```python
from build123d import *

# Parameters (mm, degrees)
SKETCH3_W           = 8
SKETCH3_H           = 8
BOSS_EXTRUDE2_DEPTH = 15.2
SKETCH4_W           = 12
SKETCH4_H           = 12
BOSS_EXTRUDE3_DEPTH = 1


with BuildPart() as part:
    # Sketch1 → Revolve1 (revolve)
    with BuildSketch(Plane(origin=(0, 0, 0), x_dir=(0, 0, -1), z_dir=(1, 0, 0))):
        Polygon((-19.2, 0), (30.8, 0), (30.8, 5), (29.8, 5), (29.8, 4), (14.6, 4), (14.6, 3.5), (13.4, 3.5), (13.4, 4), (0, 4), (0, 2.5), (-15.4, 2.5), (-15.4, 2), (-16.2, 2), (-16.2, 2.5), (-19.2, 2.5), align=None)
    revolve(axis=Axis((0, 0, 19.2), (0, 0, -1)))

    # Sketch3 → Boss-Extrude2 (add)
    with BuildSketch(Plane.XY.offset(-29.8)):
        Rectangle(SKETCH3_W, SKETCH3_H)
    extrude(amount=BOSS_EXTRUDE2_DEPTH)

    # Sketch4 → Boss-Extrude3 (add)
    with BuildSketch(Plane(origin=(0, 0, -30.8), x_dir=(-1, 0, 0), z_dir=(0, 0, -1))):
        Rectangle(SKETCH4_W, SKETCH4_H)
    extrude(amount=-BOSS_EXTRUDE3_DEPTH)


solid = part.part
```
Here's how the part is built. I have some questions about the finished solid (model axes, mm). A direction names the side the tool comes from. Round coordinates to 2 decimals unless told otherwise and drop trailing zeros. Loops run counter-clockwise (first coordinate to the right, second up) from the corner with the lowest first, then second, coordinate; pieces in that order, holes last.
1. Suppose I cut it at A-A, the plane y = 0. Please give me the cut outline in (x, z), and give its area (3 significant figures).
Answers:
outline: (-6, -30.8) - (6, -30.8) - (6, -29.8) - (4, -29.8) - (4, -14.6) - (3.5, -14.6) - (3.5, -13.4) - (4, -13.4) - (4, 0) - (2.5, 0) - (2.5, 15.4) - (2, 15.4) - (2, 16.2) - (2.5, 16.2) - (2.5, 19.2) - (-2.5, 19.2) - (-2.5, 16.2) - (-2, 16.2) - (-2, 15.4) - (-2.5, 15.4) - (-2.5, 0) - (-4, 0) - (-4, -13.4) - (-3.5, -13.4) - (-3.5, -14.6) - (-4, -14.6) - (-4, -29.8) - (-6, -29.8) - close
area: 344 mm2
2. Will these pins go through, and if not, where does the flat tip stop? pin 1 (4 mm diameter, centred on x = 1.5, z = -22, fed in from -Y); pin 2 (1.5 mm diameter, centred on x = -4, z = 13, fed in from -Y); pin 3 (5 mm diameter, centred on y = 2, z = 5, fed in from -X); pin 4 (6 mm diameter, centred on x = 0.5, y = 2.5, fed in from +Z).
Answers:
pin 1: stops at y = -4
pin 2: passes through
pin 3: stops at x = -2.5
pin 4: stops at z = 19.2
3. If I drill on probe 1 along Z at (x, y) = (-1.25, 2); probe 2 along Y at (x, z) = (2.5, -27.5); probe 3 along Z at (x, y) = (5, 1.5), over which ranges is the centre line in solid material (lowest first)?
Answers:
probe 1: z = -30.8 to 15.4, 16.2 to 19.2
probe 2: y = -4 to 4
probe 3: z = -30.8 to -29.8
4. For faces 5 (the face through (4, 0, -22)), 6 (the face through (0, -4, -22)), 7 (the face through (2, -1, 15.4)), which set-ups out of +Z, -Z, +X, -X, +Y, -Y let a thin tool reach every point of the face, with its end or its side?
Answers:
face 5: +Z, +X, +Y, -Y
face 6: +Z, +X, -X, -Y
face 7: none
5. Suppose I cut it at C-C, the plane z = -5.5. Please give me the cut outline in (x, y), and give its area (3 significant figures).
Answers:
outline: circle Ø8 at (0, 0)
area: 50.3 mm2
6. Thinking about a two-plate mould opening in Z: for faces 1 (the face through (2, 1, 16.2)), 2 (the face through (-3.6, -0.8, -14.6)), 3 (the face through (0, 0, -30.8)), 4 (the face through (-2.44, -0.54, 7.81)), which applies, released by +Z, released by -Z, zero draft, split by the parting line, or undercut?
Answers:
face 1: undercut
face 2: undercut
face 3: released by -Z
face 4: zero draft
7. Suppose I cut it at D-D, the plane z = 8. Please give me the cut outline in (x, y), and give its area (3 significant figures).
Answers:
outline: circle Ø5 at (0, 0)
area: 19.6 mm2
